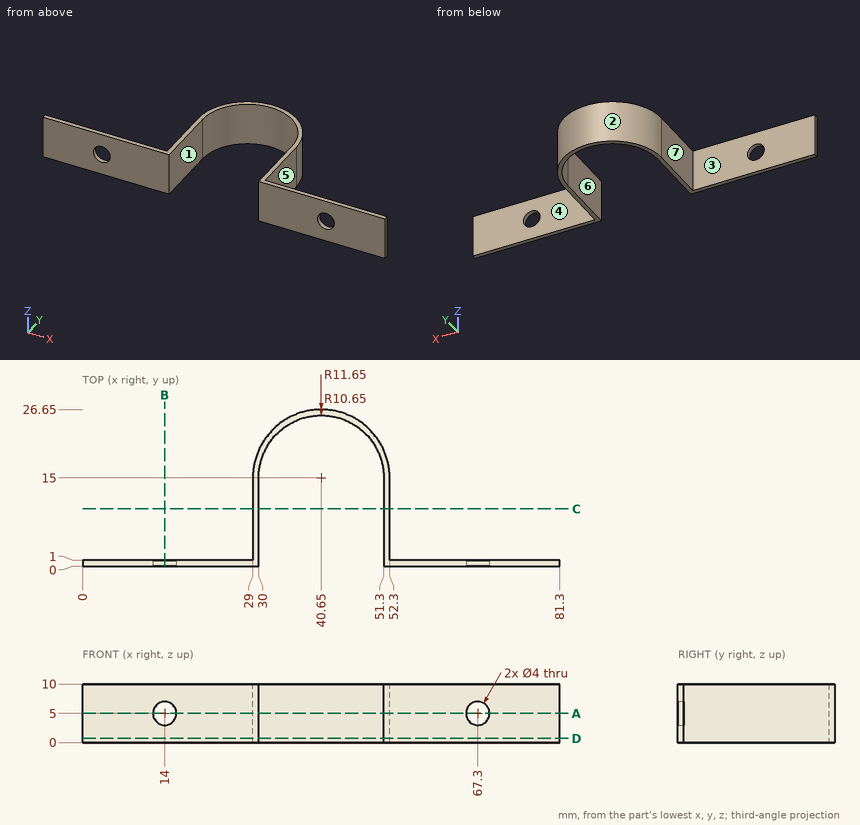
Design review of the part shown in the three views and the two pictorial views. Dimensions are in mm from the part's minimum x, y and z. A direction names the side the tool comes from. Give positions to 0.01 mm unless a question says otherwise; leave off trailing zeros. Loops run counter-clockwise (first coordinate to the right, second up) from the corner with the lowest first, then second, coordinate; pieces in that order, holes last. Notation, with made-up numbers: (-9.5, 1) -> (16.5, 1) arc R23 cw to (16.5, 9) -> close; hole circle Ø10 at (75.5, 21). An arc over 180 degrees is marked (long way). Answer as a JSON object with one key per item and string values. Group by question number.
Q1. Take a section at A-A (z = 5). Write out the cut boundary in (x, y), plus the area to 3 significant figures.
Q2. Tool access review of the marked faces 1, 2 and 3: name each direction out of +Z, -Z, +X, -X, +Y, -Y from which nothing blocks a thin tool from reaching the whole face with its end or side.
Q3. Take a section at D-D (z = 0.75). Write out the cut boundary in (x, y).
Q4. Draft analysis for pull direction X (two halves, no side actions). For the marked faces 4, 5, 6 and 7, state which applies: pulls with the +X half, pulls with the -X half, needs draft (parallel to the pull), parting line crosses it, or undercut.
Q5. Insertion check: pin 1 (3 mm diameter, centred on y = 8.5, z = 2.5, fed in from +X); pin 2 (5 mm diameter, centred on x = 67.3, z = 5, fed in from -Y); pin 3 (5 mm diameter, centred on x = 70, z = 7, fed in from +Y). Each pin has a flat end and moves straight along its axis. Give the tip position at first contact, or say it passes through.
Q6. Take a section at C-C (y = 9.75). Write out the cut boundary in (x, z).
Q7. Take a section at B-B (x = 14). Write out the cut boundary in (y, z), plus the area to 3 significant figures.
Q8. Wall thickness on line 1 along Z through (x, y) = (67.3, 0.6); line 2 along X through (y, z) = (4, 9); line 3 along Y through (x, z) = (23.5, 2): over which ranges is each line inside the solid? List them lowest first.
Answer below:
{
 "1": {"outline": "(0, 0) -> (12, 0) -> (12, 1) -> (0, 1) -> close; (16, 0) -> (30, 0) -> (30, 15) arc R10.65 cw to (51.3, 15) -> (51.3, 0) -> (65.3, 0) -> (65.3, 1) -> (52.3, 1) -> (52.3, 15) arc R11.65 ccw to (29, 15) -> (29, 1) -> (16, 1) -> close; (69.3, 0) -> (81.3, 0) -> (81.3, 1) -> (69.3, 1) -> close", "area": "115 mm2"},
 "2": {"face 1": "+Z, -Z, -Y", "face 2": "+Z, -Z, +Y", "face 3": "+Z, -Z, -X, +Y"},
 "3": {"outline": "(0, 0) -> (30, 0) -> (30, 15) arc R10.65 cw to (51.3, 15) -> (51.3, 0) -> (81.3, 0) -> (81.3, 1) -> (52.3, 1) -> (52.3, 15) arc R11.65 ccw to (29, 15) -> (29, 1) -> (0, 1) -> close"},
 "4": {"face 4": "needs draft", "face 5": "pulls with the +X half", "face 6": "undercut", "face 7": "pulls with the -X half"},
 "5": {"pin 1": "stops at x = 52.3", "pin 2": "stops at y = 0", "pin 3": "stops at y = 1"},
 "6": {"outline": "(29, 0) -> (30, 0) -> (30, 10) -> (29, 10) -> close; (51.3, 0) -> (52.3, 0) -> (52.3, 10) -> (51.3, 10) -> close"},
 "7": {"outline": "(0, 0) -> (1, 0) -> (1, 3) -> (0, 3) -> close; (0, 7) -> (1, 7) -> (1, 10) -> (0, 10) -> close", "area": "6.00 mm2"},
 "8": {"line 1": "z = 0 to 3, 7 to 10", "line 2": "x = 29 to 30, 51.3 to 52.3", "line 3": "y = 0 to 1"}
}
